from build123d import *

# Parameters (mm, degrees)
SKETCH1_W           = 30
SKETCH1_H           = 30
BOSS_EXTRUDE1_DEPTH = 350
SKETCH2_R           = 40
BOSS_EXTRUDE2_DEPTH = 10
SKETCH3_R           = 17.5
CUT_EXTRUDE1_DEPTH  = 5


with BuildPart() as part:
    # Sketch1 → Boss-Extrude1 (new, symmetric)
    with BuildSketch(Plane(origin=(0, 0, 0), x_dir=(0, 0, -1), z_dir=(1, 0, 0))):
        Rectangle(SKETCH1_W, SKETCH1_H)
    extrude(amount=BOSS_EXTRUDE1_DEPTH, both=True)

    # Sketch2 → Boss-Extrude2 (add)
    with BuildSketch(Plane(origin=(0, 15, 0), x_dir=(1, 0, 0), z_dir=(0, 1, 0))):
        with Locations(Location((303.514520503, 0, 0), (0, 0, 157.975687163))):
            Circle(SKETCH2_R)
    boss_extrude2 = extrude(amount=BOSS_EXTRUDE2_DEPTH)

    # Sketch3 → Cut-Extrude1 (cut)
    with BuildSketch(Plane(origin=(0, 25, 0), x_dir=(1, 0, 0), z_dir=(0, 1, 0))):
        with Locations(Location((303.514520503, 0, 0), (0, 0, 270))):
            Circle(SKETCH3_R)
    cut_extrude1 = extrude(amount=-CUT_EXTRUDE1_DEPTH, mode=Mode.SUBTRACT)

    # Mirror1: Boss-Extrude2, Cut-Extrude1 across plane
    add(boss_extrude2.mirror(Plane(origin=(0, 0, 0), x_dir=(0, 0, 1), z_dir=(1, 0, 0))))
    add(cut_extrude1.mirror(Plane(origin=(0, 0, 0), x_dir=(0, 0, 1), z_dir=(1, 0, 0))), mode=Mode.SUBTRACT)


solid = part.part
Verification items for the finished model (mm, model axes). A direction names the side the tool comes from. Give positions to 0.01 mm unless a question says otherwise; leave off trailing zeros. Order: outer loops, then holes, each group sorted by start corner. A loop starts at its lowest first (then second) coordinate and runs counter-clockwise, first axis right, second up. Notation, with made-up numbers: M -3.5,64.5 L 49.5,64.5 A5 cw 49.5,71.5 Z; hole C -2,-28 d8. An arc over 180 degrees is marked long. Answer as a JSON object with one key per item and string values. Group by question number.
1) Cross-section at B-B (z = -34). Enter the section's corners in (x, y), then the cut area to 3 significant figures.
2) Mould release check, pull along Z, two halves, no side actions. Record for faces 6 (the face through (-342.068, 19.93, -10.66)), 7 (the face through (-304, 20, 0)), 8 (the face through (5, -15, 0)), 9 (the face through (5, 0, 15)): released by +Z, released by -Z, zero draft, split by the parting line, or undercut.
3) Cross-section at C-C (y = -9). Enter the section's corners in (x, z).
4) Scan lines: line 1 along X through (y, z) = (21, 0); line 2 along Y through (x, z) = (-105.5, -1); line 3 along Y through (x, z) = (-315.5, -8.5). Record each from-to range of solid material in increasing order. Write a range as [from, to].
5) Cross-section at D-D (x = 0). Enter the section's corners in (y, z).
6) Depth check by flat-ended pin: pin 1 Ø17.5 at (x, z) = (298, 5.5) entering from +Y; pin 2 Ø20 at (x, z) = (-312.5, -26.5) entering from -Y; pin 3 Ø6 at (x, y) = (-157.5, -5) entering from +Z; pin 4 Ø12 at (y, z) = (17, 13) entering from -X. Enter the tip coordinate at first touch or a pass-through.
7) Cross-section at A-A (z = 0). Enter the section's corners in (x, y).
8) Access from +Z, -Z, +X, -X, +Y, -Y to the whole of each face (thin tool, end or side, straight path). Record for faces 1 (the face through (-307, 15, 28)), 2 (the face through (-302, 25, -19)), 3 (the face through (304, 20, 0)), 4 (the face through (301, 15, -27)), 5 (the face through (4, 15, 0)).
Result sheet:
{
 "1": {"outline": "M -324.59,15 L -282.44,15 L -282.44,25 L -324.59,25 Z; M 282.44,15 L 324.59,15 L 324.59,25 L 282.44,25 Z", "area": "843 mm2"},
 "2": {"face 6": "split by the parting line", "face 7": "undercut", "face 8": "zero draft", "face 9": "released by +Z"},
 "3": {"outline": "M -350,-15 L 350,-15 L 350,15 L -350,15 Z"},
 "4": {"line 1": "x = [-343.51, -321.01], [-286.01, -263.51], [263.51, 286.01], [321.01, 343.51]", "line 2": "y = [-15, 15]", "line 3": "y = [-15, 20]"},
 "5": {"outline": "M -15,-15 L 15,-15 L 15,15 L -15,15 Z"},
 "6": {"pin 1": "stops at y = 20", "pin 2": "stops at y = 15", "pin 3": "stops at z = 15", "pin 4": "stops at x = -350"},
 "7": {"outline": "M -350,-15 L 350,-15 L 350,15 L 343.51,15 L 343.51,25 L 321.01,25 L 321.01,20 L 286.01,20 L 286.01,25 L 263.51,25 L 263.51,15 L -263.51,15 L -263.51,25 L -286.01,25 L -286.01,20 L -321.01,20 L -321.01,25 L -343.51,25 L -343.51,15 L -350,15 Z"},
 "8": {"face 1": "+Z, +X, -X, -Y", "face 2": "+Z, -Z, +X, -X, +Y", "face 3": "+Y", "face 4": "-Z, +X, -X, -Y", "face 5": "+Z, -Z, +Y"}
}
